Input: part model. Units: mm. Frame: model coordinates. A direction names the side the tool comes from. Give positions to 0.01 mm unless a question says otherwise; leave off trailing zeros. Order: outer loops, then holes, each group sorted by start corner. A loop starts at its lowest first (then second) coordinate and runs counter-clockwise, first axis right, second up. Notation, with made-up numbers: (-28, 25) - (18, 25) arc R27 ccw to (18, 42) - close; hole circle Ø5 at (87, 33). An arc over 180 degrees is marked (long way). Answer in a Markdown table with one row per item. Add a question column.
1. Access query for faces 1 (the face through (20.6, -5.44, -15.43)), 2 (the face through (7, 0, 5)), 3 (the face through (-3, -0.5, 2.5)), 4 (the face through (7, -4, 6)). Directions: +Z, -Z, +X, -X, +Y, -Y. A direction counts if a zero-diameter tool reaches every point of the face in a straight line with its end or side. Return the directions, or none.
2. Contact query for flat-ended pins moving along their axis: pin 1 (5 mm diameter, centred on x = 2.5, y = -2.5, fed in from -Z); pin 2 (1.1 mm diameter, centred on y = -0.5, z = 2, fed in from -X); pin 3 (5 mm diameter, centred on x = 7, y = -0.5, fed in from +Z). Output: stop coordinate, or through.
3. Mould query, pull axis Y, two halves, no side actions, for faces 5 (the face through (13.75, 0.05, 2.46)), 6 (the face through (-4.702, -3.705, -0.614)), 7 (the face through (-5.6, -5.44, -15.43)). Classes: released by +Y, released by -Y, zero draft, split by the parting line, or undercut.
4. Section query B-B on y = -5.25. Return loops of the section in (x, z), and give its area (3 significant figures).
5. Section query D-D on z = 7. Return loops of the section in (x, y).
6. Ray query, line 1 (Y direction, x = 0, z = 1); line 2 (X direction, y = -4.5, z = -14); line 3 (Y direction, x = -9, z = 10.5). Return the intervals inside material, ascending. Write a range as [from, to].
7. Section query C-C on x = 12. Return loops of the section in (y, z).
8. Section query A-A on z = -8.5. Return loops of the section in (x, y), and give its area (3 significant figures).
```python
from build123d import *

# Parameters (mm, degrees)
SKETCH_1_R      = 1.25
EXTRUDE_1_DEPTH = 5
SKETCH_2_W      = 41
SKETCH_2_H      = 15
EXTRUDE_2_DEPTH = 3
SKETCH_4_W      = 8
SKETCH_4_H      = 16
EXTRUDE_3_DEPTH = 3
FILLET_1_R      = 3
FILLET_2_R      = 5
FILLET_3_R      = 2


with BuildPart() as part:
    # ｽｹｯﾁ1 → ﾎﾞｽ - 押し出し1 (new body)
    with BuildSketch(Plane.XY):
        with BuildLine():
            Line((-3, -4), (18, -4))
            Line((18, -4), (18, 0))
            ThreePointArc((18, 0), (17.121320344, 2.121320344), (15, 3))
            Line((15, 3), (0, 3))
            ThreePointArc((0, 3), (-2.121320344, 2.121320344), (-3, 0))
            Line((-3, 0), (-3, -4))
        make_face()
        Circle(SKETCH_1_R, mode=Mode.SUBTRACT)
        with Locations((15, 0)):
            Circle(SKETCH_1_R, mode=Mode.SUBTRACT)
    extrude(amount=EXTRUDE_1_DEPTH)

    # ｽｹｯﾁ2 → ﾎﾞｽ - 押し出し2 (add)
    with BuildSketch(Plane.XZ.offset(4)):
        with Locations((7.5, 7.5)):
            Rectangle(SKETCH_2_W, SKETCH_2_H)
    extrude(amount=EXTRUDE_2_DEPTH)

    # ｽｹｯﾁ4 → ﾎﾞｽ - 押し出し3 (add)
    with BuildSketch(Plane(origin=(0, -4, 0), x_dir=(1, 0, 0), z_dir=(0, 1, 0))):
        with Locations((-9, 8)):
            Rectangle(SKETCH_4_W, SKETCH_4_H)
        with Locations((24, 8)):
            Rectangle(SKETCH_4_W, SKETCH_4_H)
    extrude(amount=-EXTRUDE_3_DEPTH)

    # ﾌｨﾚｯﾄ1
    fillet_1_edges = [part.edges().sort_by_distance(p)[0] for p in [
        (-3, -4, 2.5),
        (18, -4, 2.5),
    ]]
    fillet(fillet_1_edges, radius=FILLET_1_R)

    # ﾌｨﾚｯﾄ2
    fillet_2_edges = [part.edges().sort_by_distance(p)[0] for p in [
        (-13, -5.5, 15),
        (28, -5.5, 15),
    ]]
    fillet(fillet_2_edges, radius=FILLET_2_R)

    # ﾌｨﾚｯﾄ3
    fillet_3_edges = [part.edges().sort_by_distance(p)[0] for p in [
        (28, -5.5, -16),
        (20, -5.414213562, -16),
        (20, -5.414213562, 0),
        (-5, -5.414213562, 0),
        (-5, -5.414213562, -16),
        (-13, -5.5, -16),
    ]]
    fillet(fillet_3_edges, radius=FILLET_3_R - 0.0001)  # a hair under: the kernel refuses the full size


solid = part.part
```
Answer:
| question | item | result |
|---|---|---|
| 1 | face 1 | -Z, +Y, -Y |
| 1 | face 2 | +Z, +X, -X, +Y |
| 1 | face 3 | +Z, -Z, -X, +Y |
| 1 | face 4 | +Z, +Y |
| 2 | pin 1 | stops at z = 0 |
| 2 | pin 2 | stops at x = -3 |
| 2 | pin 3 | stops at z = 5 |
| 3 | face 5 | undercut |
| 3 | face 6 | released by +Y |
| 3 | face 7 | zero draft |
| 4 | outline | (-13, -14) arc R2 ccw to (-11, -16) - (-7, -16) arc R2 ccw to (-5, -14) - (-5, -2) arc R2 cw to (-3, 0) - (18, 0) arc R2 cw to (20, -2) - (20, -14) arc R2 ccw to (22, -16) - (26, -16) arc R2 ccw to (28, -14) - (28, 10) arc R5 ccw to (23, 15) - (-8, 15) arc R5 ccw to (-13, 10) - close |
| 4 | area | 859 mm² |
| 5 | outline | (-13, -7) - (28, -7) - (28, -4) - (-13, -4) - close |
| 6 | line 1 | y = [-7, -1.25], [1.25, 3] |
| 6 | line 2 | x = [-13, -5], [20, 28] |
| 6 | line 3 | y = [-7, -4] |
| 7 | outline | (-7, 0) - (3, 0) - (3, 5) - (-4, 5) - (-4, 15) - (-7, 15) - close |
| 8 | outline | (-13, -7) - (-5, -7) - (-5, -3.83) arc R3 cw to (-6, -4) - (-13, -4) - close; (20, -7) - (28, -7) - (28, -4) - (21, -4) arc R3 cw to (20, -3.83) - close |
| 8 | area | 48.1 mm² |
